from build123d import *

# Parameters (mm, degrees)
SKETCH1_R           = 12.7
BOSS_EXTRUDE1_DEPTH = 165
SKETCH7_R           = 12.7
BOSS_EXTRUDE3_DEPTH = 150
SKETCH10_W          = 10
SKETCH10_H          = 15.657586021
BOSS_EXTRUDE8_DEPTH = 50
SKETCH11_R          = 1.85
CUT_EXTRUDE2_DEPTH  = 239.140019974


with BuildPart() as part:
    # Sketch1 → Boss-Extrude1 (new body)
    with BuildSketch(Plane(origin=(0, 0, 0), x_dir=(0, 0, -1), z_dir=(1, 0, 0))):
        Circle(SKETCH1_R)
    extrude(amount=BOSS_EXTRUDE1_DEPTH)

    # Sketch7 → Boss-Extrude3 (add)
    with BuildSketch(Plane(origin=(62.5, -62.5, 0), x_dir=(0.7071067811865464, 0.7071067811865488, 0), z_dir=(-0.7071067811865488, 0.7071067811865464, 0))):
        with Locations(Location((88.388347648, 0, 0), (0, 0, 90))):
            Circle(SKETCH7_R)
    extrude(amount=BOSS_EXTRUDE3_DEPTH)

    # Sketch10 → Boss-Extrude8 (add)
    with BuildSketch(Plane(origin=(-43.566017178, 43.566017178, 0), x_dir=(0, 0, 1), z_dir=(-0.7071067811865487, 0.7071067811865465, 0))):
        with Locations((-5, 88.388347649)):
            Rectangle(SKETCH10_W, SKETCH10_H)
    extrude(amount=BOSS_EXTRUDE8_DEPTH)

    # Sketch11 → Cut-Extrude2 (cut, through all)
    with BuildSketch(Plane(origin=(165, 0, 0), x_dir=(0, 0, -1), z_dir=(1, 0, 0))):
        Circle(SKETCH11_R)
    extrude(amount=-CUT_EXTRUDE2_DEPTH, mode=Mode.SUBTRACT)


solid = part.part
Source: CAD feature listing. Evaluate the final solid. Frame: model axes, mm. A direction names the side the tool comes from. Round coordinates to 2 decimals unless told otherwise and drop trailing zeros. Loops run counter-clockwise (first coordinate to the right, second up) from the corner with the lowest first, then second, coordinate; pieces in that order, holes last.
Q1. Section C-C, the plane x = 44. State how many separate pieces and enclosed holes the cut face has, plus the area to 3 significant figures.
Q2. Access query for faces 5 (the face through (1, 123, 0)), 6 (the face through (-4.03, 117.96, -5.07)), 7 (the face through (18.81, 105.94, 4.03)). Directions: +Z, -Z, +X, -X, +Y, -Y. A direction counts if a zero-diameter tool reaches every point of the face in a straight line with its end or side. Return the directions, or none.
Q3. Section B-B, the plane z = 8.5. Return loops of the section in (x, y).
Q4. Mould query, pull axis Y, two halves, no side actions, for faces 1 (the face through (81.476, 61.057, 2.753)), 2 (the face through (18.86, 105.99, -11.03)), 3 (the face through (81.34, -12.4, 2.75)), 4 (the face through (0, 0, -3)). Classes: pulls with the +Y half, pulls with the -Y half, needs draft (parallel to the pull), parting line crosses it, or undercut.
Q5. Section D-D, the plane y = 129. Return loops of the section in (x, z).
Q6. First-contact query: P1, Ø3, axis at y = 119.5, z = -1.5, coming from the -X side; P2, Ø6, axis at y = 26, z = 2, coming from the -X side; P3, Ø5, axis at x = 30.5, z = 8, coming from the +Y side. Flat tips, straight axial feed; report the tip coordinate or a pass-through.
Q7. Ray query, line 1 (Y direction, x = 53, z = 0); line 2 (Y direction, x = 101, z = 0); line 3 (X direction, y = 0, z = -2). Return the intervals inside material, ascending.
Q8. Section A-A, the plane x = 145. Return loops of the section in (y, z).
Solutions:
1. separate pieces: 2
1. enclosed holes: 1
1. area: 1,210 mm2
2. face 5: +Z, -X, +Y
2. face 6: +Z, -Z, -X
2. face 7: +Z
3. outline: (0, -9.44) - (165, -9.44) - (165, 9.44) - (128.91, 9.44) - (25.61, 112.74) - (12.26, 99.39) - (102.22, 9.44) - (0, 9.44) - close
4. face 1: undercut
4. face 2: pulls with the +Y half
4. face 3: undercut
4. face 4: needs draft
5. outline: (-15.07, -10) - (7.07, -10) - (7.07, 0) - (-15.07, 0) - close
6. P1: stops at x = -7.07
6. P2: stops at x = 78.21
6. P3: stops at y = 111.93
7. line 1: y = -12.7 to -1.85, 1.85 to 12.7, 54.04 to 89.96
7. line 2: y = -12.7 to -1.85, 1.85 to 41.96
7. line 3: x = 0 to 165
8. outline: circle Ø25.4 at (0, 0); hole circle Ø3.7 at (0, 0)
